```python
from build123d import *

# Parameters (mm, degrees)
F0_W     = 2
F0_H     = 16.0696078092
F1_DEPTH = 25
F2_SIZE  = 5
F3_SIZE  = 1
F4_T     = -2.5


with BuildPart() as f1:
    # F0 (on Top) → F1 (new body)
    with BuildSketch(Plane.XY):
        with Locations((1, 8.0348039046)):
            Rectangle(F0_W, F0_H)
        Polygon((-17.9578904063, 0), (0, 0), (0, 16.0696078092), (0, 27.5092944503), (-39.9500094354, 27.5092944503), (-39.9500094354, 0), align=None)
    extrude(amount=F1_DEPTH)

    # F2
    f2_edges = [f1.edges().sort_by_distance(p)[0] for p in [
        (0, 27.509294, 12.5),
        (-39.950009, 27.509294, 12.5),
        (-19.975005, 27.509294, 0),
        (-19.975005, 27.509294, 25),
    ]]
    chamfer(f2_edges, length=F2_SIZE)

    # F3
    f3_edges = [f1.edges().sort_by_distance(p)[0] for p in [
        (2, 16.069608, 12.5),
    ]]
    chamfer(f3_edges, length=F3_SIZE)

    # F4
    f4_openings = [f1.faces().sort_by_distance(p)[0] for p in [
        (-18.975005, 0, 12.5),
    ]]
    offset(amount=F4_T, openings=f4_openings, kind=Kind.INTERSECTION)


solid = f1.part
```
Source: CAD feature listing. Evaluate the final solid. Frame: model axes, mm. A direction names the side the tool comes from. Coordinates: 2 decimals unless noted, no trailing zeros. Order: outer loops, then holes, each group sorted by start corner. A loop starts at its lowest first (then second) coordinate and runs counter-clockwise, first axis right, second up. Notation, with made-up numbers: (43.25, 25.5) - (71.25, 25.5) arc R14 cw to (71.25, 31.5) - close; hole circle Ø2 at (-24, -3). An arc over 180 degrees is marked (long way). One line per item, written item: value.
1) Ray query, line 1 (Z direction, x = -23, y = 3); line 2 (X direction, y = 20.5, z = 3.75); line 3 (X direction, y = 5.25, z = 19.75). Return the intervals inside material, ascending. Write a range as [from, to].
Computed values:
line 1: z = [0, 2.5], [22.5, 25]
line 2: x = [-39.95, -37.45], [-2.5, 0]
line 3: x = [-39.95, -37.45], [-0.5, 2]
2) Reachability of faces 1 (the face through (0, 19, 12)), 2 (the face through (-0.5, 7, 12)), 3 (the face through (-19.7, 24.97, 2.46)) from +Z, -Z, +X, -X, +Y, -Y: full face, straight path, thin tool, end or side. Return the list, or none.
Computed values:
face 1: +Z, -Z, +X, +Y
face 2: -Y
face 3: -Z, +X, -X, +Y
3) Cut plane D-D on y = 23. Output: boundary loops of the cut face in (x, z), plus the area to 3 significant figures.
Computed values:
outline: (-39.46, 0.49) - (-0.49, 0.49) - (-0.49, 24.51) - (-39.46, 24.51) - close; hole (-35.92, 4.03) - (-4.03, 4.03) - (-4.03, 20.97) - (-35.92, 20.97) - close
area: 395 mm^2
4) Mould query, pull axis X, two halves, no side actions, for faces 4 (the face through (2, 7, 12)), 5 (the face through (-35.707, 23.217, 12.36)), 6 (the face through (-19.7, 24.97, 22.54)). Classes: released by +X, released by -X, zero draft, split by the parting line, or undercut.
Computed values:
face 4: released by +X
face 5: undercut
face 6: zero draft
5) Contact query for flat-ended pins moving along their axis: pin 1 (12 mm diameter, centred on x = -4, z = 10, fed in from -Y); pin 2 (10.5 mm diameter, centred on x = -16.5, z = 11.5, fed in from -Y); pin 3 (10 mm diameter, centred on x = -8.5, z = 15, fed in from -Y); pin 4 (1 mm diameter, centred on x = -23, z = 5.5, fed in from -Y). Output: stop coordinate, or through.
Computed values:
pin 1: stops at y = 0
pin 2: stops at y = 25.01
pin 3: stops at y = 22.47
pin 4: stops at y = 23.97
6) Cut plane C-C on x = -8.5. Output: boundary loops of the cut face in (y, z).
Computed values:
outline: (0, 0) - (22.51, 0) - (27.51, 5) - (27.51, 20) - (22.51, 25) - (0, 25) - (0, 22.5) - (21.47, 22.5) - (25.01, 18.96) - (25.01, 6.04) - (21.47, 2.5) - (0, 2.5) - close
7) Cut plane B-B on z = 9. Output: boundary loops of the cut face in (x, y).
Computed values:
outline: (-39.95, 0) - (-37.45, 0) - (-37.45, 21.47) - (-33.91, 25.01) - (-6.04, 25.01) - (-2.5, 21.47) - (-2.5, 13.57) - (-0.5, 13.57) - (-0.5, 0) - (2, 0) - (2, 15.07) - (1, 16.07) - (0, 16.07) - (0, 22.51) - (-5, 27.51) - (-34.95, 27.51) - (-39.95, 22.51) - close
8) Cut plane A-A on y = 9.75. Output: boundary loops of the cut face in (x, z).
Computed values:
outline: (-39.95, 0) - (2, 0) - (2, 25) - (-39.95, 25) - close; hole (-37.45, 2.5) - (-0.5, 2.5) - (-0.5, 22.5) - (-37.45, 22.5) - close
